Here's how the part is built. I have some questions about the finished solid (model axes, mm). Face numbers are marked on the shaded views. A direction names the side the tool comes from. Coordinates: 2 decimals unless noted, no trailing zeros. Order: outer loops, then holes, each group sorted by start corner. A loop starts at its lowest first (then second) coordinate and runs counter-clockwise, first axis right, second up.
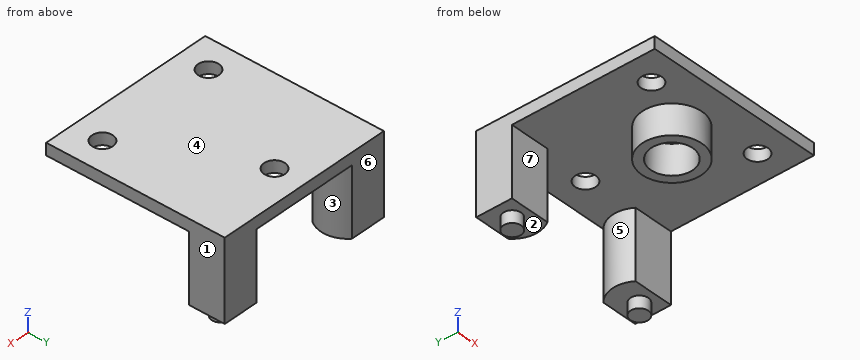
```python
from build123d import *

# Parameters (mm, degrees)
SKETCH1_W           = 30
SKETCH1_H           = 30
BOSS_EXTRUDE1_DEPTH = 2
BOSS_EXTRUDE3_DEPTH = 11.5
SKETCH3_R           = 1.5
BOSS_EXTRUDE4_DEPTH = 2
SKETCH4_R           = 5
SKETCH4_R_2         = 3.5
BOSS_EXTRUDE5_DEPTH = 5
SKETCH5_R           = 1.75
CUT_EXTRUDE1_DEPTH  = 3


with BuildPart() as part:
    # Sketch1 → Boss-Extrude1 (new body)
    with BuildSketch(Plane.XY):
        with Locations((14.990081794, 9.125005221)):
            Rectangle(SKETCH1_W, SKETCH1_H)
    extrude(amount=BOSS_EXTRUDE1_DEPTH)

    # Sketch2 → Boss-Extrude3 (add)
    with BuildSketch(Plane(origin=(0, 0, 0), x_dir=(-1, 0, 0), z_dir=(0, 0, -1))):
        with BuildLine():
            Line((0.009918206, 24.125005221), (0.009918206, 18.125005221))
            Line((0.009918206, 18.125005221), (-6.682350101, 18.125005221))
            ThreePointArc((-6.682350101, 18.125005221), (-7.494065902, 21.253655407), (-6.009921446, 24.125005221))
            Line((-6.009921446, 24.125005221), (0.009918206, 24.125005221))
        make_face()
    boss_extrude3 = extrude(amount=BOSS_EXTRUDE3_DEPTH)

    # Sketch3 → Boss-Extrude4 (add)
    with BuildSketch(Plane(origin=(0, 0, -11.5), x_dir=(-1, 0, 0), z_dir=(0, 0, -1))):
        with Locations((-3.00000162, 20.74999914)):
            Circle(SKETCH3_R)
    boss_extrude4 = extrude(amount=BOSS_EXTRUDE4_DEPTH)

    # Mirror1: Boss-Extrude3, Boss-Extrude4 across plane
    add(boss_extrude3.mirror(Plane(origin=(14.990081794, 0, 0), x_dir=(0, 0, 1), z_dir=(1, 0, 0))))
    add(boss_extrude4.mirror(Plane(origin=(14.990081794, 0, 0), x_dir=(0, 0, 1), z_dir=(1, 0, 0))))

    # Sketch4 → Boss-Extrude5 (add)
    with BuildSketch(Plane(origin=(0, 0, 0), x_dir=(-1, 0, 0), z_dir=(0, 0, -1))):
        with Locations((-13.707999, 3.46499688)):
            Circle(SKETCH4_R)
        with Locations((-13.707999, 3.46499688)):
            Circle(SKETCH4_R_2, mode=Mode.SUBTRACT)
    extrude(amount=BOSS_EXTRUDE5_DEPTH)

    # Sketch5 → Cut-Extrude1 (cut, through all)
    with BuildSketch(Plane(origin=(0, 0, 0), x_dir=(-1, 0, 0), z_dir=(0, 0, -1))):
        with Locations((-24.990081794, -0.874994779)):
            Circle(SKETCH5_R)
        with Locations((-4.990081794, -0.874994779)):
            Circle(SKETCH5_R)
        with Locations((-14.990081794, 19.125005221)):
            Circle(SKETCH5_R)
    extrude(amount=-CUT_EXTRUDE1_DEPTH, mode=Mode.SUBTRACT)


solid = part.part
```
Q1. I need wall thicknesses on L1, parallel to Z at x = 26.5, y = 4.75; L2, parallel to X at y = 19.5, z = -9.5; L3, parallel to Y at x = 14.5, z = -2.75. Which ranges of each line are inside material? Lowest first, please.
Q2. If we section it at B-B on y = 20.25: Write out the boundary of the cut face in (x, z).
Q3. Will these pins go through, and if not, where does the flat tip stop? pin 1 (7.5 mm diameter, centred on x = 26, z = -8, fed in from -Y) (3 decimals); pin 2 (15 mm diameter, centred on x = 22.5, y = 16, fed in from -Z); pin 3 (11 mm diameter, centred on x = 16, y = 1.5, fed in from -Z); pin 4 (5.5 mm diameter, centred on x = 4.99, y = -0.87, fed in from -Z).
Q4. If we section it at A-A on z = -8: Write out the boundary of the cut face in (x, y) (3 decimals).
Q5. If we section it at C-C on z = -3.5: Write out the boundary of the cut face in (x, y) (3 decimals), then the cut area to 3 significant figures.
Q6. We'd pull the mould along X, two halves only. Please class the marked faces 1, 2, 3 and 4: pulls with the +X half, pulls with the -X half, needs draft (parallel to the pull), parting line crosses it, or undercut.
Q7. If we section it at D-D on x = 25: Write out the boundary of the cut face in (y, z) (3 decimals), then the cut area to 3 significant figures.
Q8. For the marked faces 5, 6 and 7, which set-ups out of +Z, -Z, +X, -X, +Y, -Y let a thin tool reach every point of the face, with its end or its side?
Reply:
1. L1: z = 0 to 2
1. L2: x = -0.01 to 7.35, 22.63 to 29.99
1. L3: y = -1.47 to 0.06, 6.87 to 8.4
2. outline: (-0.01, -11.5) - (1.59, -11.5) - (1.59, -13.5) - (4.41, -13.5) - (4.41, -11.5) - (7.49, -11.5) - (7.49, 0) - (13.65, 0) - (13.65, 2) - (-0.01, 2) - close; (16.33, 0) - (22.49, 0) - (22.49, -11.5) - (25.57, -11.5) - (25.57, -13.5) - (28.39, -13.5) - (28.39, -11.5) - (29.99, -11.5) - (29.99, 2) - (16.33, 2) - close
3. pin 1: stops at y = 18.125
3. pin 2: stops at z = -13.5
3. pin 3: stops at z = -5
3. pin 4: stops at z = 0
4. outline: (-0.01, 18.125) - (6.682, 18.125) arc R4.522 ccw to (6.01, 24.125) - (-0.01, 24.125) - close; (23.298, 18.125) - (29.99, 18.125) - (29.99, 24.125) - (23.97, 24.125) arc R4.522 ccw to start
5. outline: (-0.01, 18.125) - (6.682, 18.125) arc R4.522 ccw to (6.01, 24.125) - (-0.01, 24.125) - close; circle Ø10 at (13.708, 3.465); (23.298, 18.125) - (29.99, 18.125) - (29.99, 24.125) - (23.97, 24.125) arc R4.522 ccw to start; hole circle Ø7 at (13.708, 3.465)
5. area: 126 mm2
6. face 1: pulls with the +X half
6. face 2: undercut
6. face 3: undercut
6. face 4: needs draft
7. outline: (-5.875, 0) - (-2.625, 0) - (-2.625, 2) - (-5.875, 2) - close; (0.875, 0) - (18.125, 0) - (18.125, -11.5) - (24.125, -11.5) - (24.125, 2) - (0.875, 2) - close
7. area: 122 mm2
8. face 5: -Z
8. face 6: +Z, -Z, +X, -X, +Y
8. face 7: -Z, +X, -X, -Y
